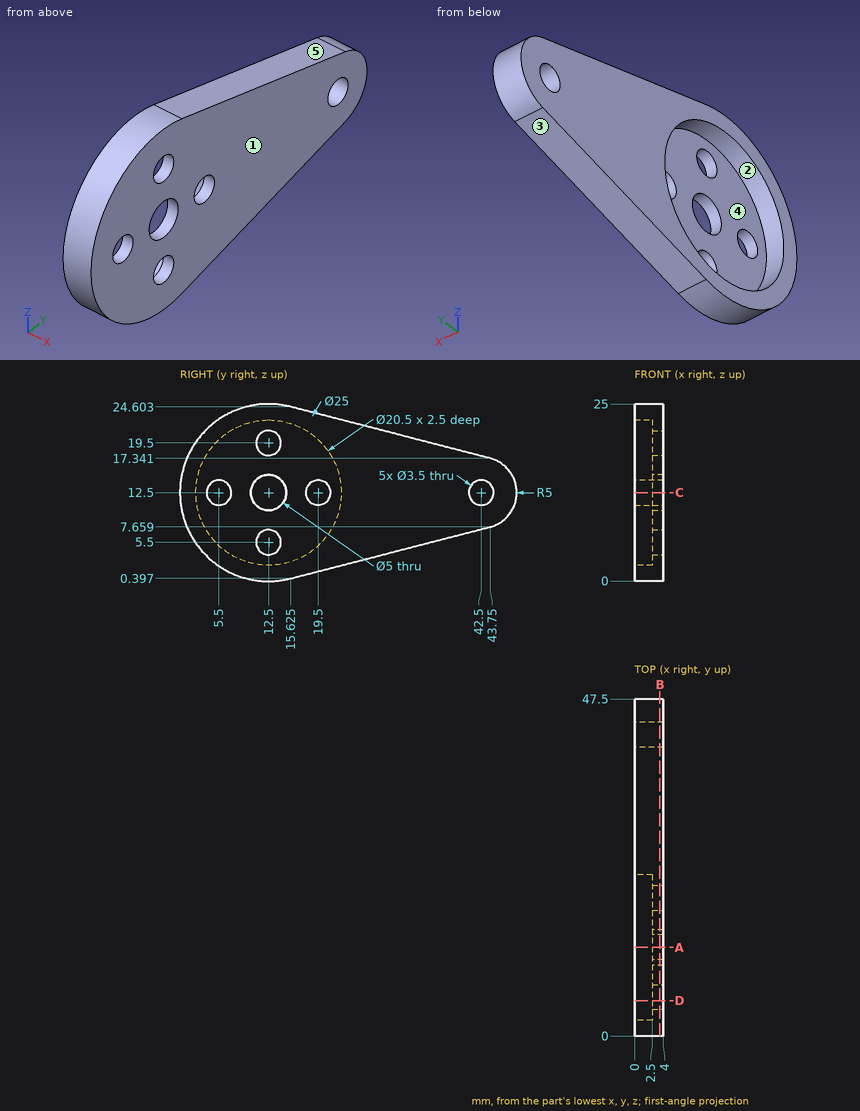
Source: three-view drawing plus pictorial views. Frame: mm from the lowest corner of the part. A direction names the side the tool comes from. Give positions to 0.01 mm unless a question says otherwise; leave off trailing zeros. Order: outer loops, then holes, each group sorted by start corner. A loop starts at its lowest first (then second) coordinate and runs counter-clockwise, first axis right, second up. Notation, with made-up numbers: M 30,-8.75 L 74,-8.75 A26 ccw 74,13.25 Z; hole C 33.25,40.5 d3. An arc over 180 degrees is marked long. Return JSON: item names as keys, results as strings.
1) Section query B-B on x = 3.55. Count the separate pieces of the cut face and the enclosed holes in it.
Taken from the geometry:
{"separate pieces": "1", "enclosed holes": "6"}
2) Section query C-C on z = 12.5. Output: boundary loops of the cut face in (x, y).
Taken from the geometry:
{"outline": "M 0,0 L 4,0 L 4,3.75 L 2.5,3.75 L 2.5,2.25 L 0,2.25 Z; M 0,22.75 L 2.5,22.75 L 2.5,21.25 L 4,21.25 L 4,40.75 L 0,40.75 Z; M 0,44.25 L 4,44.25 L 4,47.5 L 0,47.5 Z; M 2.5,7.25 L 4,7.25 L 4,10 L 2.5,10 Z; M 2.5,15 L 4,15 L 4,17.75 L 2.5,17.75 Z"}
3) Contact query for flat-ended pins moving along their axis: pin 1 (4.5 mm diameter, centred on y = 5.5, z = 12.5, fed in from -X); pin 2 (3 mm diameter, centred on y = 12.5, z = 5.5, fed in from +X); pin 3 (1 mm diameter, centred on x = 2.5, y = 5.5, fed in from +Z). Output: stop coordinate, or through.
Taken from the geometry:
{"pin 1": "stops at x = 2.5", "pin 2": "passes through", "pin 3": "stops at z = 23.18"}
4) Section query D-D on y = 5. Output: boundary loops of the cut face in (x, z).
Taken from the geometry:
{"outline": "M 0,2.5 L 4,2.5 L 4,10.82 L 2.5,10.82 L 2.5,5.51 L 0,5.51 Z; M 0,19.49 L 2.5,19.49 L 2.5,14.18 L 4,14.18 L 4,22.5 L 0,22.5 Z"}
5) Line query: L1, parallel to Z at x = 3, y = 12.5; L2, parallel to Y at x = 1.9, z = 11.5; L3, parallel to X at y = 13, z = 9.25. Output: solid intervals per line, ascending. Write a range as [from, to].
Taken from the geometry:
{"L1": "z = [0, 3.75], [7.25, 10], [15, 17.75], [21.25, 25]", "L2": "y = [0.04, 2.3], [22.7, 41.06], [43.94, 47.4]", "L3": "x = [2.5, 4]"}
6) Access query for the marked faces 4 and 5. Directions: +Z, -Z, +X, -X, +Y, -Y. A direction counts if a zero-diameter tool reaches every point of the face in a straight line with its end or side. Return the directions, or none.
Taken from the geometry:
{"face 4": "-X", "face 5": "+Z, +X, -X, +Y"}
7) Mould query, pull axis Y, two halves, no side actions, for the marked faces 1, 2 and 3. Classes: released by +Y, released by -Y, zero draft, split by the parting line, or undercut.
Taken from the geometry:
{"face 1": "zero draft", "face 2": "undercut", "face 3": "released by +Y"}
8) Section query A-A on y = 12.5. Output: boundary loops of the cut face in (x, z).
Taken from the geometry:
{"outline": "M 0,0 L 4,0 L 4,3.75 L 2.5,3.75 L 2.5,2.25 L 0,2.25 Z; M 0,22.75 L 2.5,22.75 L 2.5,21.25 L 4,21.25 L 4,25 L 0,25 Z; M 2.5,7.25 L 4,7.25 L 4,10 L 2.5,10 Z; M 2.5,15 L 4,15 L 4,17.75 L 2.5,17.75 Z"}
